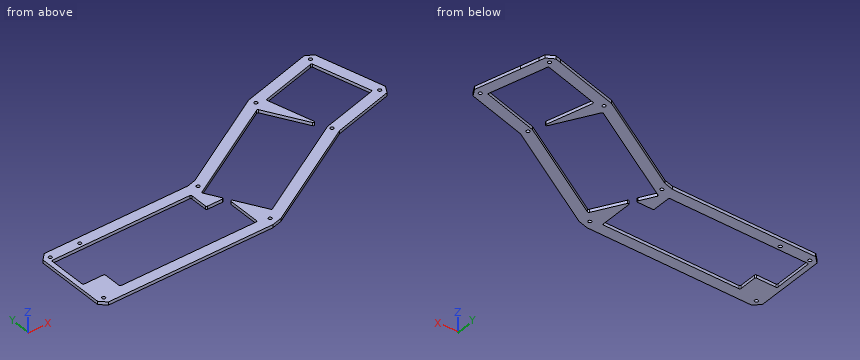
from build123d import *

# Parameters (mm, degrees)
ESQUISSE1_R        = 1.6
BOSS_EXTRU_1_DEPTH = 3


with BuildPart() as part:
    # Esquisse1 → Boss.-Extru.1 (new body)
    with BuildSketch(Plane.XY):
        Polygon((-75.988646329, 50.585106383), (-96.375082906, 50.585106383), (-102.253762562, 44.706426727), (-102.253762562, 35.79522772), (-102.253762562, -22.536213961), (-96.375082906, -28.414893617), (63.866204609, -28.414893617), (73.57783127, -25.812671096), (178.129773206, 34.550420725), (236.676113061, 50.237865209), (240.83296731, 57.437747969), (229.542938833, 99.572707865), (224.885316316, 116.95519174), (223.46218398, 122.391704558), (216.287606244, 126.561599525), (210.79963, 125.091100722), (147.636911389, 108.166701279), (52.055735868, 52.982883862), (43.107108491, 50.585106383), align=None)
        with Locations((-95.753762562, 44.085106383)):
            Circle(ESQUISSE1_R, mode=Mode.SUBTRACT)
        with Locations((-66.988646329, 44.085106383)):
            Circle(ESQUISSE1_R, mode=Mode.SUBTRACT)
        with Locations((-95.753762562, -21.914893617)):
            Circle(ESQUISSE1_R, mode=Mode.SUBTRACT)
        with Locations((49.263745973, 45.505477252)):
            Circle(ESQUISSE1_R, mode=Mode.SUBTRACT)
        with Locations((67.039694146, -20.835264486)):
            Circle(ESQUISSE1_R, mode=Mode.SUBTRACT)
        with Locations((175.637377655, 40.567595866)):
            Circle(ESQUISSE1_R, mode=Mode.SUBTRACT)
        with Locations((234.393639901, 56.355573542)):
            Circle(ESQUISSE1_R, mode=Mode.SUBTRACT)
        with Locations((217.363403759, 120.120565138)):
            Circle(ESQUISSE1_R, mode=Mode.SUBTRACT)
        with Locations((150.12930694, 102.149526137)):
            Circle(ESQUISSE1_R, mode=Mode.SUBTRACT)
        with BuildLine():
            Line((-97.753762562, 39.085106383), (-97.753762562, 2.085106383))
            ThreePointArc((-97.753762562, 2.085106383), (-97.460869343, 1.377999602), (-96.753762562, 1.085106383))
            Line((-96.753762562, 1.085106383), (-77.753762562, 1.085106383))
            ThreePointArc((-77.753762562, 1.085106383), (-77.046655781, 0.792213164), (-76.753762562, 0.085106383))
            Line((-76.753762562, 0.085106383), (-76.753762562, -16.914893617))
            ThreePointArc((-76.753762562, -16.914893617), (-76.460869343, -17.622000398), (-75.753762562, -17.914893617))
            Line((-75.753762562, -17.914893617), (56.011353671, -17.914893617))
            ThreePointArc((56.011353671, -17.914893617), (56.718460453, -17.622000398), (57.011353671, -16.914893617))
            Line((57.011353671, -16.914893617), (57.011353671, 14.621004768))
            ThreePointArc((57.011353671, 14.621004768), (57.752534626, 15.586930594), (58.877379075, 15.121004768))
            Line((58.877379075, 15.121004768), (74.527293708, -11.98544251))
            ThreePointArc((74.527293708, -11.98544251), (75.134500067, -12.451368337), (75.893319112, -12.351467914))
            Line((75.893319112, -12.351467914), (174.076924484, 44.334863077))
            Line((174.076924484, 44.334863077), (228.528734589, 58.925181621))
            ThreePointArc((228.528734589, 58.925181621), (229.135940948, 59.391107448), (229.235841371, 60.149926493))
            Line((229.235841371, 60.149926493), (214.741974845, 114.241772765))
            ThreePointArc((214.741974845, 114.241772765), (214.276049019, 114.848979124), (213.517229973, 114.948879546))
            Line((213.517229973, 114.948879546), (159.425383701, 100.45501302))
            ThreePointArc((159.425383701, 100.45501302), (158.818177343, 99.989087194), (158.71827692, 99.230268149))
            Line((158.71827692, 99.230268149), (170.271736655, 56.112169417))
            ThreePointArc((170.271736655, 56.112169417), (169.688494261, 54.929470839), (168.439785425, 55.353350371))
            Line((168.439785425, 55.353350371), (146.120215143, 94.011980101))
            ThreePointArc((146.120215143, 94.011980101), (145.513008785, 94.477905928), (144.75418974, 94.378005505))
            Line((144.75418974, 94.378005505), (46.893319112, 37.878005505))
            ThreePointArc((46.893319112, 37.878005505), (46.427393286, 37.270799147), (46.527293708, 36.511980101))
            Line((46.527293708, 36.511980101), (54.567977999, 22.585106383))
            ThreePointArc((54.567977999, 22.585106383), (54.567977999, 21.585106383), (53.701952595, 21.085106383))
            Line((53.701952595, 21.085106383), (39.011353671, 21.085106383))
            ThreePointArc((39.011353671, 21.085106383), (38.30424689, 21.377999602), (38.011353671, 22.085106383))
            Line((38.011353671, 22.085106383), (38.011353671, 39.085106383))
            ThreePointArc((38.011353671, 39.085106383), (37.718460453, 39.792213164), (37.011353671, 40.085106383))
            Line((37.011353671, 40.085106383), (-96.753762562, 40.085106383))
            ThreePointArc((-96.753762562, 40.085106383), (-97.460869343, 39.792213164), (-97.753762562, 39.085106383))
        make_face(mode=Mode.SUBTRACT)
    extrude(amount=BOSS_EXTRU_1_DEPTH)


solid = part.part
Design review of the part built by this model. Coordinates are the model's own, in mm. Coordinates: 2 decimals unless noted, no trailing zeros. Loops run counter-clockwise (first coordinate to the right, second up) from the corner with the lowest first, then second, coordinate; pieces in that order, holes last.
Item 1: Add section A-A (x = -24.5). Write out the cut boundary in (y, z), and give its area (3 significant figures).
Completed:
outline: (-28.41, 0) - (-17.91, 0) - (-17.91, 3) - (-28.41, 3) - close; (40.09, 0) - (50.59, 0) - (50.59, 3) - (40.09, 3) - close
area: 63.0 mm2
Item 2: Wall thickness on L1, parallel to Y at x = -67, z = 1.75; L2, parallel to Y at x = -10.5, z = 0.5; L3, parallel to X at y = -3, z = 1.55: over which ranges is each line inside the solid? List them lowest first.
Completed:
L1: y = -28.41 to -17.91, 40.09 to 42.49, 45.69 to 50.59
L2: y = -28.41 to -17.91, 40.09 to 50.59
L3: x = -102.25 to -76.75, 57.01 to 69.34, 92.09 to 113.09
Item 3: Add section C-C (x = 182). Write out the cut boundary in (y, z), and give its area (3 significant figures).
Completed:
outline: (35.59, 0) - (46.46, 0) - (46.46, 3) - (35.59, 3) - close; (106.5, 0) - (117.37, 0) - (117.37, 3) - (106.5, 3) - close
area: 65.2 mm2
Item 4: Add section B-B (y = 73.5). Write out the cut boundary in (x, z).
Completed:
outline: (87.59, 0) - (108.59, 0) - (108.59, 3) - (87.59, 3) - close; (157.96, 0) - (165.61, 0) - (165.61, 3) - (157.96, 3) - close; (225.66, 0) - (236.53, 0) - (236.53, 3) - (225.66, 3) - close
Item 5: Clearance check with flat-ended pins moving along their axes: pin 1 (1 mm diameter, centred on x = 89, z = 1, fed in from +Y); pin 2 (3.5 mm diameter, centred on x = 234.39, y = 56.36, fed in from +Z); pin 3 (1.5 mm diameter, centred on x = -7, z = 1, fed in from +Y); pin 4 (1 mm diameter, centred on y = 87, z = 1.5, fed in from +X). State where each tip first meets the part, or that it passes through.
Completed:
pin 1: stops at y = 74.6
pin 2: stops at z = 3
pin 3: stops at y = 50.59
pin 4: stops at x = 233.05
Item 6: Add section D-D (z = 2.15). Give the number of separate pieces and of enclosed holes in the cut face, and give its area (3 significant figures).
Completed:
separate pieces: 1
enclosed holes: 10
area: 9,490 mm2
